Can you work these out from the model? Positions are in its coordinate system, mm. Round coordinates to 2 decimals unless told otherwise and drop trailing zeros. Loops run counter-clockwise (first coordinate to the right, second up) from the corner with the lowest first, then second, coordinate; pieces in that order, holes last. Notation, with made-up numbers: (49, 78.25) -> (93, 78.25) arc R18 ccw to (93, 99.25) -> close; hole circle Ø9 at (2, -20.5). An arc over 180 degrees is marked (long way). Use a Markdown table: item, result.
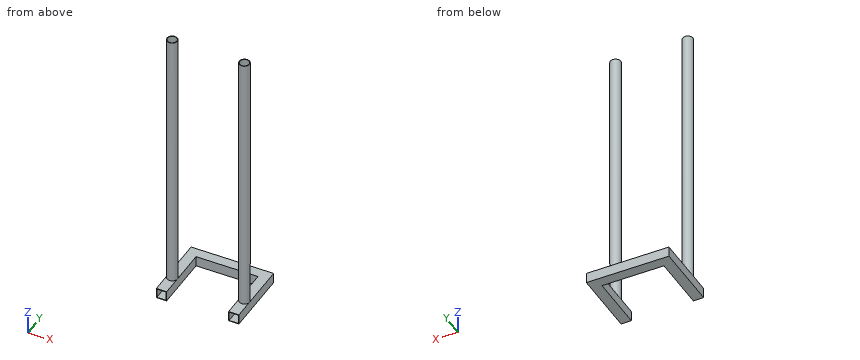
from build123d import *

# Parameters (mm, degrees)
SKETCH1_R             = 12.7
SKETCH1_R_2           = 11.4554
BOSS_EXTRUDE1_DEPTH   = 660.4
BOSS_EXTRUDE1_2_DEPTH = 660.4
BOSS_EXTRUDE2_DEPTH   = 25.4
SHELL1_START          = -24.1554
SHELL1_DEPTH          = 22.9108


# Read off the part's stored shape, not the designer's step: Shell1
with BuildPart() as part:
    # Sketch1 → Boss-Extrude1 (new body)
    with BuildSketch(Plane.XY):
        with Locations((-88.9, 0)):
            Circle(SKETCH1_R)
        with Locations((-88.9, 0)):
            Circle(SKETCH1_R_2, mode=Mode.SUBTRACT)
    extrude(amount=BOSS_EXTRUDE1_DEPTH)



with BuildPart() as body_2:
    # Sketch1 → Boss-Extrude1 2 (new body)
    with BuildSketch(Plane.XY):
        with Locations(Location((88.9, 0, 0), (0, 0, 180))):
            Circle(SKETCH1_R)
        with Locations(Location((88.9, 0, 0), (0, 0, 180))):
            Circle(SKETCH1_R_2, mode=Mode.SUBTRACT)
    extrude(amount=BOSS_EXTRUDE1_2_DEPTH)


with BuildPart() as part_1:
    add(part.part)

    add(body_2.part)  # Boss-Extrude2 merges body 2
    # Sketch2 → Boss-Extrude2 (add)
    with BuildSketch(Plane(origin=(0, 0, 0), x_dir=(-1, 0, 0), z_dir=(0, 0, -1))):
        Polygon((101.6, 0), (101.6, 114.3), (-101.6, 114.3), (-101.6, 0), (-101.6, -50.8), (-76.2, -50.8), (-76.2, 0), (-76.2, 88.9), (76.2, 88.9), (76.2, 0), (76.2, -50.8), (101.6, -50.8), align=None)
    extrude(amount=BOSS_EXTRUDE2_DEPTH)

    # Shell1 outline → Shell1 (cut)
    with BuildSketch(Plane.XY.offset(SHELL1_START)):
        Polygon((-100.3554, 113.0554), (-100.3554, -50.8), (-77.4446, -50.8), (-77.4446, 90.1446), (77.4446, 90.1446), (77.4446, -50.8), (100.3554, -50.8), (100.3554, 113.0554), align=None)
    extrude(amount=SHELL1_DEPTH, mode=Mode.SUBTRACT)


solid = part_1.part
1. I want a section at B-B (x = 6.5). Please give me the cut outline in (y, z), plus the area to 3 significant figures.
Answer sheet:
| item | result |
|---|---|
| outline | (88.9, -25.4) -> (114.3, -25.4) -> (114.3, 0) -> (88.9, 0) -> close; hole (90.14, -24.16) -> (113.06, -24.16) -> (113.06, -1.24) -> (90.14, -1.24) -> close |
| area | 120 mm² |
2. I want a section at A-A (z = 179.5). Please give me the cut outline in (x, y), plus the area to 3 significant figures.
Answer sheet:
| item | result |
|---|---|
| outline | circle Ø25.4 at (-88.9, 0); circle Ø25.4 at (88.9, 0); hole circle Ø22.91 at (-88.9, 0); hole circle Ø22.91 at (88.9, 0) |
| area | 189 mm² |
3. Will these pins go through, and if not, where does the flat tip stop? pin 1 Ø20.5 at (x, z) = (-33.5, -18.5) entering from -Y; pin 2 Ø20.5 at (x, y) = (-88.9, 0) entering from +Z.
Answer sheet:
| item | result |
|---|---|
| pin 1 | stops at y = 88.9 |
| pin 2 | stops at z = 0 |
4. I want a section at C-C (x = 88.9). Please give me the cut outline in (y, z), plus the area to 3 significant figures.
Answer sheet:
| item | result |
|---|---|
| outline | (-50.8, -25.4) -> (114.3, -25.4) -> (114.3, 0) -> (12.7, 0) -> (12.7, 660.4) -> (11.46, 660.4) -> (11.46, 0) -> (-11.46, 0) -> (-11.46, 660.4) -> (-12.7, 660.4) -> (-12.7, 0) -> (-50.8, 0) -> (-50.8, -1.24) -> (113.06, -1.24) -> (113.06, -24.16) -> (-50.8, -24.16) -> close |
| area | 2,080 mm² |
5. I need wall thicknesses on line 1 (X direction, y = 0.5, z = 546.5); line 2 (Y direction, x = 88.9, z = 307.5); line 3 (X direction, y = 5, z = 75). Which ranges of each line are inside material? Lowest first, please.
Answer sheet:
| item | result |
|---|---|
| line 1 | x = -101.59 to -100.34, -77.46 to -76.21, 76.21 to 77.46, 100.34 to 101.59 |
| line 2 | y = -12.7 to -11.46, 11.46 to 12.7 |
| line 3 | x = -100.57 to -99.21, -78.59 to -77.23, 77.23 to 78.59, 99.21 to 100.57 |
